from build123d import *

# Parameters (mm, degrees)
BOSS_EXTRUDE1_DEPTH = 2.54
SHELL1_START        = 6.4516
SHELL1_OUTLINE_W    = 2.3368
SHELL1_OUTLINE_H    = 75.9968
SHELL1_DEPTH        = 520.4968
SHELL1_START_2      = 0.1016
SHELL1_2_OUTLINE_W  = 2.3368
SHELL1_2_OUTLINE_H  = 25.1968
SHELL1_2_DEPTH      = 533.1968
SHELL1_START_3      = 50.9016
SHELL1_3_OUTLINE_W  = 2.3368
SHELL1_3_OUTLINE_H  = 6.35
SHELL1_3_DEPTH      = 50.5968
SHELL1_START_4      = 241.4016
SHELL1_4_OUTLINE_W  = 2.3368
SHELL1_4_OUTLINE_H  = 6.35
SHELL1_4_DEPTH      = 50.5968
SHELL1_START_5      = 431.9016
SHELL1_5_OUTLINE_W  = 2.3368
SHELL1_5_OUTLINE_H  = 6.35
SHELL1_5_DEPTH      = 50.5968


# Read off the part's stored shape, not the designer's step: Shell1
with BuildPart() as part:
    # Sketch1 → Boss-Extrude1 (new body)
    with BuildSketch(Plane(origin=(0, 0, 0), x_dir=(1, 0, 0), z_dir=(0, 1, 0))):
        Polygon((292.1, -76.2), (292.1, -82.55), (241.3, -82.55), (241.3, -76.2), (101.6, -76.2), (101.6, -82.55), (50.8, -82.55), (50.8, -76.2), (0, -76.2), (0, -50.8), (6.35, -50.8), (6.35, -25.4), (0, -25.4), (0, 0), (533.4, 0), (533.4, -25.4), (527.05, -25.4), (527.05, -50.8), (533.4, -50.8), (533.4, -76.2), (482.6, -76.2), (482.6, -82.55), (431.8, -82.55), (431.8, -76.2), align=None)
    extrude(amount=BOSS_EXTRUDE1_DEPTH)

    # Shell1 outline → Shell1 (cut)
    with BuildSketch(Plane.YZ.offset(SHELL1_START)):
        with Locations((1.27, 38.1)):
            Rectangle(SHELL1_OUTLINE_W, SHELL1_OUTLINE_H)
    extrude(amount=SHELL1_DEPTH, mode=Mode.SUBTRACT)

    # Shell1 2 outline → Shell1 2 (cut)
    with BuildSketch(Plane.YZ.offset(SHELL1_START_2)):
        with Locations((1.27, 63.5)):
            Rectangle(SHELL1_2_OUTLINE_W, SHELL1_2_OUTLINE_H)
        with Locations((1.27, 12.7)):
            Rectangle(SHELL1_2_OUTLINE_W, SHELL1_2_OUTLINE_H)
    extrude(amount=SHELL1_2_DEPTH, mode=Mode.SUBTRACT)

    # Shell1 3 outline → Shell1 3 (cut)
    with BuildSketch(Plane.YZ.offset(SHELL1_START_3)):
        with Locations((1.27, 79.2734)):
            Rectangle(SHELL1_3_OUTLINE_W, SHELL1_3_OUTLINE_H)
    extrude(amount=SHELL1_3_DEPTH, mode=Mode.SUBTRACT)

    # Shell1 4 outline → Shell1 4 (cut)
    with BuildSketch(Plane.YZ.offset(SHELL1_START_4)):
        with Locations((1.27, 79.2734)):
            Rectangle(SHELL1_4_OUTLINE_W, SHELL1_4_OUTLINE_H)
    extrude(amount=SHELL1_4_DEPTH, mode=Mode.SUBTRACT)

    # Shell1 5 outline → Shell1 5 (cut)
    with BuildSketch(Plane.YZ.offset(SHELL1_START_5)):
        with Locations((1.27, 79.2734)):
            Rectangle(SHELL1_5_OUTLINE_W, SHELL1_5_OUTLINE_H)
    extrude(amount=SHELL1_5_DEPTH, mode=Mode.SUBTRACT)


solid = part.part
Read the model definition and answer for the solid it produces. Units are mm, in the model's axes. Round coordinates to 2 decimals unless told otherwise and drop trailing zeros. Write each loop counter-clockwise with the first axis right and the second up, starting at its lowest first coordinate (ties: lowest second). Pieces come first, ordered by that corner, then holes. Notation, with made-up numbers: (87, 5) - (143, 5) arc R32 ccw to (143, 40) - close; hole circle Ø6 at (-34, -7). An arc over 180 degrees is marked (long way). One line per question, with ' | ' between items. Start each with the question number.
1. Section A-A (x = 126) is taken. Determine the outline of the cut face in (y, z), and give its area (3 significant figures).
2. Section B-B (z = 43) is taken. Determine the outline of the cut face in (x, y), and give its area (3 significant figures).
3. Each of these flat-tipped pins is pushed along its axis until it touches: pin 1 (1.3 mm diameter, centred on x = 529.5, y = 1.5, fed in from +Z); pin 2 (1.5 mm diameter, centred on y = 0.5, z = 42, fed in from +X); pin 3 (1.3 mm diameter, centred on y = 1.5, z = 79.5, fed in from -X). Where does it stop, or does it pass through?
Filled in:
1) outline: (0, 0) - (2.54, 0) - (2.54, 76.2) - (0, 76.2) - close; hole (0.1, 0.1) - (2.44, 0.1) - (2.44, 76.1) - (0.1, 76.1) - close | area: 16.0 mm²
2) outline: (6.35, 0) - (527.05, 0) - (527.05, 2.54) - (6.35, 2.54) - close; hole (6.45, 0.1) - (526.95, 0.1) - (526.95, 2.44) - (6.45, 2.44) - close | area: 106 mm²
3) pin 1: z = 76.2 | pin 2: x = 527.05 | pin 3: x = 50.8
